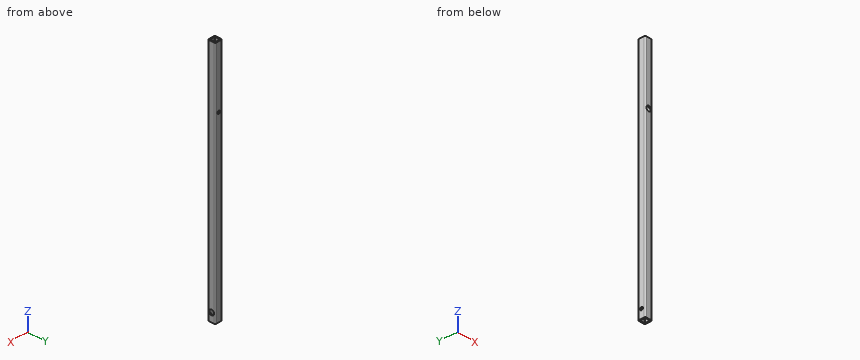
```python
from build123d import *

# Parameters (mm, degrees)
F1_DEPTH = 622.3
F2_R     = 3.683
F3_DEPTH = 47.498
F4_R     = 6.35
F5_DEPTH = 4.064
F6_R     = 3.683
F7_DEPTH = 25.4
F8_R     = 6.35
F9_DEPTH = 8.636


with BuildPart() as f1:
    # F0 (on Top) → F1 (new body)
    with BuildSketch(Plane.XY):
        with BuildLine():
            ThreePointArc((0, 3.175), (0.929936, 0.929936), (3.175, 0))
            Line((3.175, 0), (15.875, 0))
            ThreePointArc((15.875, 0), (18.120064, 0.929936), (19.05, 3.175))
            Line((19.05, 3.175), (19.05, 15.875))
            ThreePointArc((19.05, 15.875), (18.120064, 18.120064), (15.875, 19.05))
            Line((15.875, 19.05), (3.175, 19.05))
            ThreePointArc((3.175, 19.05), (0.929936, 18.120064), (0, 15.875))
            Line((0, 15.875), (0, 3.175))
        make_face()
        with BuildLine():
            ThreePointArc((3.048, 14.986), (3.34558, 15.70442), (4.064, 16.002))
            Line((4.064, 16.002), (14.986, 16.002))
            ThreePointArc((14.986, 16.002), (15.70442, 15.70442), (16.002, 14.986))
            Line((16.002, 14.986), (16.002, 4.064))
            ThreePointArc((16.002, 4.064), (15.70442, 3.34558), (14.986, 3.048))
            Line((14.986, 3.048), (4.064, 3.048))
            ThreePointArc((4.064, 3.048), (3.34558, 3.34558), (3.048, 4.064))
            Line((3.048, 4.064), (3.048, 14.986))
        make_face(mode=Mode.SUBTRACT)
    extrude(amount=F1_DEPTH)

    # F2 (on Right) → F3 (cut)
    with BuildSketch(Plane.YZ):
        with Locations((9.525, 22.225)):
            Circle(F2_R)
    extrude(amount=F3_DEPTH, mode=Mode.SUBTRACT)

    # F4 (on face) → F5 (cut)
    with BuildSketch(Plane.YZ.offset(19.05)):
        with Locations((9.525, 22.225)):
            Circle(F4_R)
    extrude(amount=-F5_DEPTH, mode=Mode.SUBTRACT)

    # F6 (on Front) → F7 (cut)
    with BuildSketch(Plane.XZ):
        with Locations((9.525, 465.328)):
            Circle(F6_R)
    extrude(amount=-F7_DEPTH, mode=Mode.SUBTRACT)

    # F8 (on face) → F9 (cut)
    with BuildSketch(Plane.XZ):
        with Locations((9.525, 465.328)):
            Circle(F8_R)
    extrude(amount=-F9_DEPTH, mode=Mode.SUBTRACT)


solid = f1.part
```
Source: CAD feature listing. Evaluate the final solid. Frame: model axes, mm. Coordinates: 2 decimals unless noted, no trailing zeros. Order: outer loops, then holes, each group sorted by start corner. A loop starts at its lowest first (then second) coordinate and runs counter-clockwise, first axis right, second up. Notation, with made-up numbers: (72.5, 49) - (104.5, 49) arc R36 ccw to (104.5, 87) - close; hole circle Ø7 at (89.25, 34.5). An arc over 180 degrees is marked (long way). One line per item, written item: value.
1) Contact query for a flat-ended pin moving along its axis: pin 1 (4.5 mm diameter, centred on y = 9.525, z = 22.225, fed in from +X). Output: stop coordinate, or through.
Computed values:
pin 1: passes through
2) Cut plane B-B on z = 445.5. Output: boundary loops of the cut face in (x, y) (3 decimals), plus the area to 3 significant figures.
Computed values:
outline: (0, 3.175) arc R3.175 ccw to (3.175, 0) - (15.875, 0) arc R3.175 ccw to (19.05, 3.175) - (19.05, 15.875) arc R3.175 ccw to (15.875, 19.05) - (3.175, 19.05) arc R3.175 ccw to (0, 15.875) - close; hole (3.048, 4.064) arc R1.016 ccw to (4.064, 3.048) - (14.986, 3.048) arc R1.016 ccw to (16.002, 4.064) - (16.002, 14.986) arc R1.016 ccw to (14.986, 16.002) - (4.064, 16.002) arc R1.016 ccw to (3.048, 14.986) - close
area: 187 mm^2
3) Cut plane A-A on x = 9.25. Output: boundary loops of the cut face in (y, z).
Computed values:
outline: (0, 0) - (3.05, 0) - (3.05, 458.98) - (0, 458.98) - close; (0, 471.67) - (3.05, 471.67) - (3.05, 622.3) - (0, 622.3) - close; (16, 0) - (19.05, 0) - (19.05, 461.66) - (16, 461.66) - close; (16, 469) - (19.05, 469) - (19.05, 622.3) - (16, 622.3) - close
4) Ray query, line 1 (X direction, y = 12.5, z = 63); line 2 (X direction, y = 3.5, z = 364). Return the intervals inside material, ascending. Write a range as [from, to].
Computed values:
line 1: x = [0, 3.05], [16, 19.05]
line 2: x = [0, 3.22], [15.83, 19.05]
5) Cut plane C-C on y = 10. Output: boundary loops of the cut face in (x, z), plus the area to 3 significant figures.
Computed values:
outline: (0, 0) - (3.05, 0) - (3.05, 18.57) - (0, 18.57) - close; (0, 25.88) - (3.05, 25.88) - (3.05, 622.3) - (0, 622.3) - close; (16, 0) - (19.05, 0) - (19.05, 15.89) - (16, 15.89) - close; (16, 28.56) - (19.05, 28.56) - (19.05, 622.3) - (16, 622.3) - close
area: 3,730 mm^2
